Can you work these out from the drawing? Everything is in mm from the part's minimum corner. Coordinates: 2 decimals unless noted, no trailing zeros. Write each loop counter-clockwise with the first axis right and the second up, starting at its lowest first coordinate (ties: lowest second). Pieces come first, ordered by that corner, then holes. Notation, with made-up numbers: (1, 33.25) - (38, 33.25) arc R20 cw to (38, 70.25) - close; hole circle Ø11 at (44.25, -2). An arc over 180 degrees is marked (long way). One line per question, with ' | ' between items. Start each with the question number.
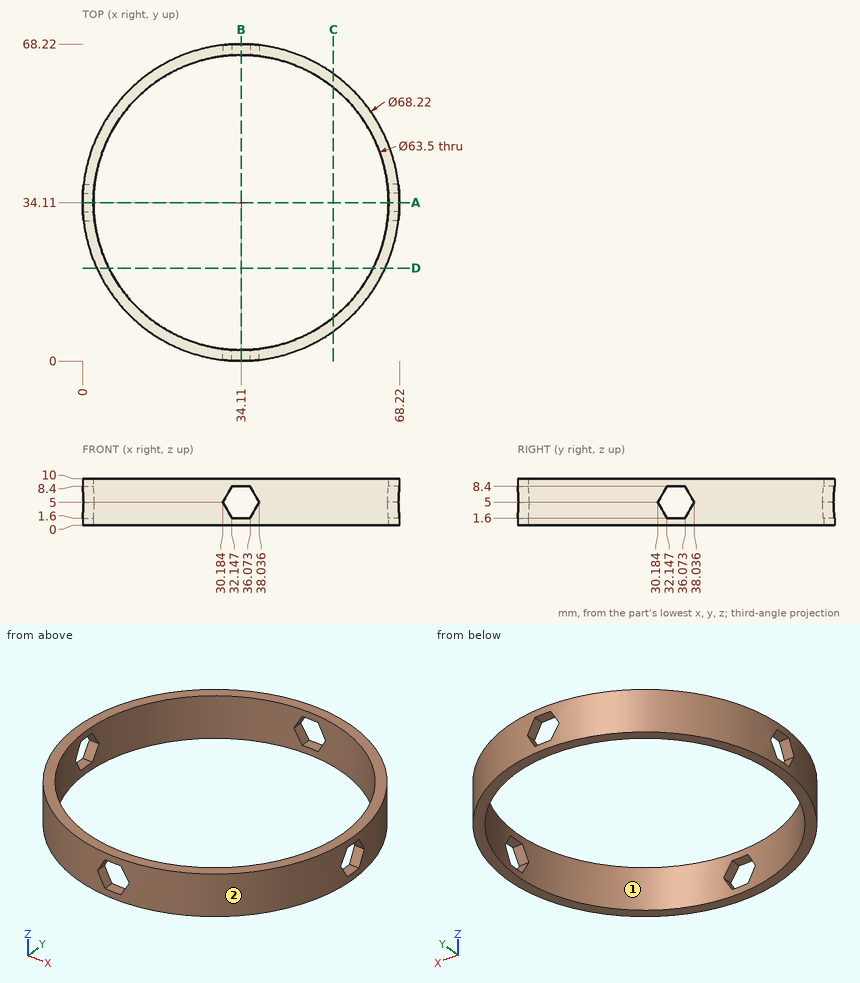
(1) I'm going to push flat-ended pins straight in: pin 1 (4 mm diameter, centred on y = 50, z = 8.5, fed in from -X); pin 2 (3 mm diameter, centred on y = 24.5, z = 2.5, fed in from -X); pin 3 (5 mm diameter, centred on y = 40, z = 3.5, fed in from -X). Where does each tip first touch, or does it pass through?
(2) If we section it at A-A on y = 34.11: List the corners of the cut face in (x, z) for me.
(3) If we section it at C-C on x = 54: List the corners of the cut face in (y, z) for me, plus the area to 3 significant figures.
(4) If I drill on probe 1 along X at (y, z) = (39.5, 5); probe 2 along Y at (x, z) = (36.5, 9.25); probe 3 along X at (y, z) = (27, 6), over which ranges is the centre line in solid material (lowest first)?
(5) If we mould it in two halves opening along X, with no side actions, what happens to the marked faces 1 and 2? For each: +X half, -X half, draft (parallel to the pull), parting line (faces both ways), or undercut.
(6) If we section it at D-D on y = 20: List the corners of the cut face in (x, z) for me, plus the area to 3 significant figures.
Values:
1) pin 1: x = 2.96 | pin 2: x = 0.98 | pin 3: x = 0.17
2) outline: (0, 0) - (2.36, 0) - (2.36, 1.6) - (0, 1.6) - close; (0, 8.4) - (2.36, 8.4) - (2.36, 10) - (0, 10) - close; (65.86, 0) - (68.22, 0) - (68.22, 1.6) - (65.86, 1.6) - close; (65.86, 8.4) - (68.22, 8.4) - (68.22, 10) - (65.86, 10) - close
3) outline: (6.4, 0) - (9.36, 0) - (9.36, 10) - (6.4, 10) - close; (58.86, 0) - (61.82, 0) - (61.82, 10) - (58.86, 10) - close | area: 59.3 mm2
4) probe 1: 0.43 to 2.82, 65.4 to 67.79 | probe 2: 0.08 to 2.45, 65.77 to 68.14 | probe 3: 0.75 to 3.17, 65.05 to 67.47
5) face 1: undercut | face 2: parting line
6) outline: (3.06, 0) - (5.67, 0) - (5.67, 10) - (3.06, 10) - close; (62.55, 0) - (65.16, 0) - (65.16, 10) - (62.55, 10) - close | area: 52.2 mm2
